from build123d import *

# Parameters (mm, degrees)
SKETCH2_R           = 1.925
BOSS_EXTRUDE1_DEPTH = 5
SKETCH2_3_R         = 1.925
BOSS_EXTRUDE2_DEPTH = 5


with BuildPart() as part:
    # Sketch2 → Boss-Extrude1 (new body)
    with BuildSketch(Plane(origin=(0, 0, 0), x_dir=(1, 0, 0), z_dir=(0, 1, 0))):
        with BuildLine():
            ThreePointArc((0, 5), (-5, 0), (0, -5))
            Line((0, -5), (30, -2.5))
            ThreePointArc((30, -2.5), (32.5, 0), (30, 2.5))
            Line((30, 2.5), (0, 5))
        make_face()
        Circle(SKETCH2_R, mode=Mode.SUBTRACT)
    extrude(amount=BOSS_EXTRUDE1_DEPTH)

    # Sketch2_3 → Boss-Extrude2 (add)
    with BuildSketch(Plane(origin=(0, 0, 0), x_dir=(1, 0, 0), z_dir=(0, 1, 0))):
        with BuildLine():
            Line((0.827586207, 4.931034483), (0, 5))
            ThreePointArc((0, 5), (-5, 0), (0, -5))
            Line((0, -5), (0.827586207, -4.931034483))
            ThreePointArc((0.827586207, -4.931034483), (3.816931427, -3.229711207), (5, 0))
            ThreePointArc((5, 0), (3.816931427, 3.229711207), (0.827586207, 4.931034483))
        make_face()
        Circle(SKETCH2_3_R, mode=Mode.SUBTRACT)
    extrude(amount=-BOSS_EXTRUDE2_DEPTH)


solid = part.part
Could you check a few things on this model? Use its own coordinates, in mm. Give positions to 0.01 mm unless a question says otherwise; leave off trailing zeros. Order: outer loops, then holes, each group sorted by start corner. A loop starts at its lowest first (then second) coordinate and runs counter-clockwise, first axis right, second up. Notation, with made-up numbers: (-38.5, 78) - (-28.5, 78) arc R23 cw to (-28.5, 106) - close; hole circle Ø2 at (-27.5, 53). An arc over 180 degrees is marked (long way). One line per item, written item: value. Start each with the question number.
1. Imagine slicing it at C-C on z = 3. List the corners of the cut face in (x, y) for me, plus the area to 3 significant figures.
2. If I drill on probe 1 along X at (y, z) = (1.3, 0) (3 decimals); probe 2 along X at (y, z) = (-0.25, 0) (3 decimals), over which ranges is the centre line in solid material (lowest first)?
3. Imagine slicing it at B-B on y = -3.75. List the corners of the cut face in (x, z) for me (3 decimals), plus the area to 3 significant figures.
4. Imagine slicing it at D-D on x = 29.5. List the corners of the cut face in (y, z) for me, plus the area to 3 significant figures.
5. Imagine slicing it at A-A on z = 1.5. List the corners of the cut face in (x, y) for me.
6. For P1, Ø1, axis at x = 11, y = 0, coming from the -Z side (3 decimals); P2, Ø2, axis at x = 8.5, y = 4, coming from the +Z side (3 decimals); P3, Ø3.5, axis at x = 0, z = 0, coming from the +Y side, each with a flat end and sliding along its axis, tell me the tip position at first contact or that it passes through.
Values:
1. outline: (-4, -5) - (4, -5) - (4, 0) - (24, 0) - (24, 5) - (-4, 5) - close
1. area: 180 mm²
2. probe 1: -5 to -1.925, 1.925 to 32.5
2. probe 2: -5 to -1.925, 1.925 to 5
3. outline: (0, -5) - (0.828, -4.931) arc R5 ccw to (0.828, 4.931) - (0, 5) arc R5 ccw to start; hole circle Ø3.85 at (0, 0)
3. area: 66.9 mm²
4. outline: (0, -2.54) - (5, -2.54) - (5, 2.54) - (0, 2.54) - close
4. area: 25.4 mm²
5. outline: (-4.77, -5) - (-1.21, -5) - (-1.21, 5) - (-4.77, 5) - close; (1.21, -5) - (4.77, -5) - (4.77, 0) - (32, 0) - (32, 5) - (1.21, 5) - close
6. P1: z = -4.125
6. P2: z = 4.375
6. P3: through
